```python
from build123d import *

# Parameters (mm, degrees)
SKETCH_1_W          = 13
SKETCH_1_H          = 160
EXTRUDE_1_DEPTH     = 3
SKETCH_2_W          = 3
SKETCH_2_H          = 160
EXTRUDE_2_DEPTH     = 135
SKETCH_3_W          = 13
SKETCH_3_H          = 138
EXTRUDE_3_DEPTH     = 3
SKETCH_4_W          = 13
SKETCH_4_H          = 138
EXTRUDE_4_DEPTH     = 3
CUT_EXTRUDE_1_DEPTH = 14


with BuildPart() as part:
    # 草圖1 → 填料-伸長1 (new body)
    with BuildSketch(Plane.XY):
        with Locations((-15.144058005, -60.964912281)):
            Rectangle(SKETCH_1_W, SKETCH_1_H)
    extrude(amount=EXTRUDE_1_DEPTH)

    # 草圖2 → 填料-伸長2 (add)
    with BuildSketch(Plane.XY.offset(3)):
        with Locations((-10.144058005, -60.964912281)):
            Rectangle(SKETCH_2_W, SKETCH_2_H)
    extrude(amount=EXTRUDE_2_DEPTH)

    # 草圖3 → 填料-伸長3 (add)
    with BuildSketch(Plane.XZ.offset(140.964912281)):
        with Locations((-15.144058005, 69)):
            Rectangle(SKETCH_3_W, SKETCH_3_H)
    extrude(amount=EXTRUDE_3_DEPTH)

    # 草圖4 → 填料-伸長4 (add)
    with BuildSketch(Plane(origin=(0, 19.035087719, 0), x_dir=(1, 0, 0), z_dir=(0, 1, 0))):
        with Locations((-15.144058005, -69)):
            Rectangle(SKETCH_4_W, SKETCH_4_H)
    extrude(amount=EXTRUDE_4_DEPTH)

    # 草圖5 → 除料-伸長1 (cut, through all)
    with BuildSketch(Plane(origin=(-8.644058005, 0, 0), x_dir=(0, 0, -1), z_dir=(1, 0, 0))):
        Polygon((-108, -76.964912281), (-108, -44.964912281), (-138, -56.100441006), (-138, -143.964912281), (-108, -143.964912281), (-108, -108.964912281), (-77.999803751, -120.099912281), (-77.999803751, -65.829912281), align=None)
        Polygon((-138, 22.035087719), (-138, -1.829383555), (-108, -12.964912281), (-108, 22.035087719), align=None)
    extrude(amount=-CUT_EXTRUDE_1_DEPTH, mode=Mode.SUBTRACT)


solid = part.part
```
Model file for the job. Use its own axes, mm. A direction names the side the tool comes from. Coordinates: 2 decimals unless noted, no trailing zeros. Write each loop counter-clockwise with the first axis right and the second up, starting at its lowest first coordinate (ties: lowest second). Pieces come first, ordered by that corner, then holes. Notation, with made-up numbers: (54.5, 79.25) - (67.5, 79.25) arc R10 cw to (67.5, 90.25) - close; hole circle Ø11 at (33, 70). An arc over 180 degrees is marked (long way). Use a Markdown table: item, result. Add a question column.
Item 1: Band-saw the part on C-C, the plane y = -5. Write the cut outline in (x, z).
Item 2: Two-plate mould, pull along Y, no slides. Class faces 1 (the face through (-8.644, -62, 55)), 2 (the face through (-10.12, -71.32, 92.79)), 3 (the face through (-10.123, -50.455, 122.79)), 4 (the face through (-11.644, -62, 55)): pulls with the +Y half, pulls with the -Y half, needs draft (parallel to the pull), parting line crosses it, or undercut.
Item 3: 3-axis set-ups, long thin cutter, end or side, ignore diameter. For faces 5 (the face through (-10.123, -114.454, 93.21)), 6 (the face through (-11, -130, 108)), 7 (the face through (-17, -140.965, 56)), 8 (the face through (-11, 7, 108)): which of +Z, -Z, +X, -X, +Y, -Y reach the whole face in a straight line?
Item 4: Band-saw the part on D-D, the plane z = 89.5. Write the cut outline in (x, y).
Item 5: Band-saw the part on A-A, the plane z = 72.5. Write the cut outline in (x, y), and give its area (3 significant figures).
Item 6: Drop flat-ended pins along their axis: pin 1 (2.5 mm diameter, centred on x = -10.5, y = -87.5, fed in from +Z); pin 2 (5 mm diameter, centred on x = -17.5, y = -32.5, fed in from +Z); pin 3 (1 mm diameter, centred on x = -10.5, z = 121.5, fed in from +Y); pin 4 (5 mm diameter, centred on x = -18, y = -90, fed in from -Z). Give the stop position or say it passes through.
Item 7: Band-saw the part on B-B, the plane x = -19. Write the cut outline in (y, z).
Item 8: Drill centre lines: line 1 along Y through (x, z) = (-14.25, 84); line 2 along Z through (x, y) = (-17.75, -24); line 3 along Z through (x, y) = (-9.25, -95). Where is each one in solid material? Low to high.
A:
| question | item | result |
|---|---|---|
| 1 | outline | (-21.64, 0) - (-8.64, 0) - (-8.64, 108) - (-11.64, 108) - (-11.64, 3) - (-21.64, 3) - close; (-11.64, 129.46) - (-8.64, 129.46) - (-8.64, 138) - (-11.64, 138) - close |
| 2 | face 1 | needs draft |
| 2 | face 2 | undercut |
| 2 | face 3 | pulls with the -Y half |
| 2 | face 4 | undercut |
| 3 | face 5 | +X, -X |
| 3 | face 6 | +Z, +X, -X, -Y |
| 3 | face 7 | +Z, -X |
| 3 | face 8 | +X, -X, +Y |
| 4 | outline | (-21.64, -143.96) - (-8.64, -143.96) - (-8.64, -115.83) - (-11.64, -115.83) - (-11.64, -140.96) - (-21.64, -140.96) - close; (-21.64, 19.04) - (-11.64, 19.04) - (-11.64, -70.1) - (-8.64, -70.1) - (-8.64, 22.04) - (-21.64, 22.04) - close |
| 5 | outline | (-21.64, -143.96) - (-8.64, -143.96) - (-8.64, 22.04) - (-21.64, 22.04) - (-21.64, 19.04) - (-11.64, 19.04) - (-11.64, -140.96) - (-21.64, -140.96) - close |
| 5 | area | 558 mm² |
| 6 | pin 1 | stops at z = 78 |
| 6 | pin 2 | stops at z = 3 |
| 6 | pin 3 | stops at y = -7.77 |
| 6 | pin 4 | stops at z = 0 |
| 7 | outline | (-143.96, 0) - (22.04, 0) - (22.04, 108) - (19.04, 108) - (19.04, 3) - (-140.96, 3) - (-140.96, 108) - (-143.96, 108) - close |
| 8 | line 1 | y = -143.96 to -140.96, 19.04 to 22.04 |
| 8 | line 2 | z = 0 to 3 |
| 8 | line 3 | z = 0 to 78 |
